Part model, mm, in its own coordinate system. Face numbers are marked on the shaded views. A direction names the side the tool comes from. Coordinates: 2 decimals unless noted, no trailing zeros. Loops run counter-clockwise (first coordinate to the right, second up) from the corner with the lowest first, then second, coordinate; pieces in that order, holes last. Notation, with made-up numbers: (75.5, 20) -> (119.5, 20) arc R27 ccw to (119.5, 41) -> close; hole circle Ø3 at (-19.75, -9). An arc over 180 degrees is marked (long way). Use one line per item in the form item = value. Start each with the question number.
(1) Mould opens along Y. For the marked faces 1 and 2 say: +Y half, -Y half, draft (parallel to the pull), parting line (faces both ways), or undercut.
(2) Pin check, flat tips, straight feed: P1, Ø1.1, axis at y = 5.5, z = -14, coming from the +X side; P2, Ø10, axis at x = -48, y = -1, coming from the +Z side; P3, Ø1.5, axis at x = -63.5, z = -2, coming from the -Y side. Stop position of each tip, or through.
(3) Drill centre lines: L1, parallel to Y at x = -4, z = 0; L2, parallel to Z at x = -91.75, y = 0; L3, parallel to Z at x = -60, y = 0. Where is each one in solid material? Low to high. Write a range as [from, to].
(4) Band-saw the part on A-A on x = -62. Give the cut face in (y, z), then the cut area to 3 significant figures.
(5) 3-axis set-ups, long thin cutter, end or side, ignore diameter. For the marked faces 3 and 4: which of +Z, -Z, +X, -X, +Y, -Y reach the whole face in a straight line?
Autodesk Inventor part; units mm, degrees
ref_plane "YZ Plane" through (0, 0, 0) normal (1, 0, 0) x (0, 1, 0)
ref_plane "XZ Plane" through (0, 0, 0) normal (0, 1, 0) x (-1, 0, 0)
ref_plane "XY Plane" through (0, 0, 0) normal (0, 0, 1) x (1, 0, 0)
sketch "Náčrt1" plane through (0, 0, 0) normal (0, 0, 1) x (1, 0, 0)
  line L0 (0, 0) -> (-100, 0)
  line L1 (-100, 0) -> (-100, 11)
  line L2 (-100, 11) -> (-20.578, 11)
  line L3 (-20.578, 11) -> (-12, 15)
  line L4 (-12, 15) -> (0, 15)
  line L5 (0, 15) -> (0, 0)
  dimension "d2" = 22
  dimension "d3" = 30
  dimension "d4" = 12
  dimension "d5" = 25
  dimension "d6" = 100
revolve "Rotace1" add sketch "Náčrt1" angle 360 about axis through (0, 0, 0) along (-1, 0, 0)
hole "Díra1" at (0, 0, 0) direction (-1, 0, 0) diameter 22.38 depth 14 tip angle 118
hole "Díra2" at (0, 0, 0) direction (-1, 0, 0) diameter 19.2 depth 75 tip angle 118
hole "Díra3" at (-100, 0, 0) direction (1, 0, 0) diameter 8.92 depth 12 tip angle 118
chamfer "Zkosení1" distance 6 angle 30 1 edges at (-100, -11, 0) measured on face at (-47.052, 10.8576, 1.7645)
sketch "Náčrt2" plane through (0, 0, 0) normal (1, 0, 0) x (0, 0, -1)
  circle A0 centre (16, 0) radius 2.6
  point P0 (0, 0)
  dimension "d40" = 16
  dimension "d41" = 5.2
extrude "Vysunutí1" cut sketch "Náčrt2" against normal blind 5
pattern_circular "Kruhové pole1" count 18 over 360 about axis through (-6, 0, 0) along (1, 0, 0) of "Vysunutí1"
chamfer "Zkosení2" distance 0.5 angle 45 1 edges at (0, 0, 11.19)
properties part number "Head02" material "ETG 100"
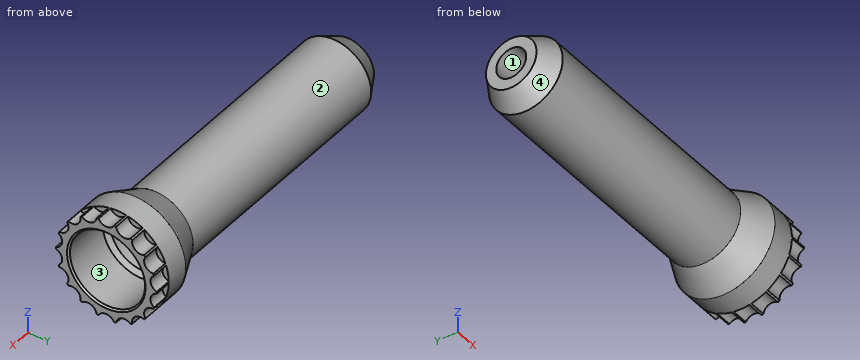
A:
q1.face_1 = undercut
q1.face_2 = parting line
q2.P1 = -5
q2.P2 = 11
q2.P3 = -10.93
q3.L1 = [-15, -11.19], [11.19, 15]
q3.L2 = [-11, -4.46], [4.46, 11]
q3.L3 = [-11, -9.6], [9.6, 11]
q4.outline = circle Ø22 at (0, 0); hole circle Ø19.2 at (0, 0)
q4.area = 90.6 mm²
q5.face_3 = +X
q5.face_4 = -X
